Here's how the part is built. I have some questions about the finished solid (model axes, mm). A direction names the side the tool comes from. Round coordinates to 2 decimals unless told otherwise and drop trailing zeros. Order: outer loops, then holes, each group sorted by start corner. A loop starts at its lowest first (then second) coordinate and runs counter-clockwise, first axis right, second up. Notation, with made-up numbers: M 7.5,-3 L 28.5,-3 A10 ccw 28.5,11 Z; hole C -29,54.25 d1. An arc over 180 degrees is marked long. Write each question's results on one line, items separated by ' | '. Start each with the question number.
```python
from build123d import *

# Parameters (mm, degrees)
SKETCH1_R                 = 24
BOSS_EXTRUDE1_DEPTH       = 3.8
SKETCH2_R                 = 18.7
BOSS_EXTRUDE2_DEPTH       = 4.5
SKETCH3_R                 = 1
CUT_EXTRUDE1_DEPTH        = 4.5
SKETCH4_R                 = 13.6
CUT_EXTRUDE2_DEPTH        = 35.941236383
SKETCH5_R                 = 40
BOSS_EXTRUDE3_DEPTH       = 17.4
SKETCH6_R                 = 32.9
CUT_EXTRUDE6_DEPTH        = 12.4
CUT_EXTRUDE7_START        = -12.4
SKETCH7_R                 = 13.6
CUT_EXTRUDE7_DEPTH        = 12.4
M2X0_4_TAPPED_HOLE1_D     = 1.6
M2X0_4_TAPPED_HOLE1_DEPTH = 5
M2X0_4_TAPPED_HOLE1_TIP   = 0.480688495


with BuildPart() as part:
    # Sketch1 → Boss-Extrude1 (new body)
    with BuildSketch(Plane.XY):
        with Locations(Location((0, 0, 0), (0, 0, 180))):
            Circle(SKETCH1_R)
    extrude(amount=BOSS_EXTRUDE1_DEPTH)

    # Sketch2 → Boss-Extrude2 (add)
    with BuildSketch(Plane.XY.offset(3.8)):
        Circle(SKETCH2_R)
    extrude(amount=BOSS_EXTRUDE2_DEPTH)

    # Sketch3 → Cut-Extrude1 (cut)
    with BuildSketch(Plane.XY.offset(3.8)):
        with Locations((0, 22.2)):
            Circle(SKETCH3_R)
    extrude(amount=-CUT_EXTRUDE1_DEPTH, mode=Mode.SUBTRACT)

    # Sketch4 → Cut-Extrude2 (cut, through all)
    with BuildSketch(Plane.XY.offset(8.3)):
        Circle(SKETCH4_R)
    extrude(amount=-CUT_EXTRUDE2_DEPTH, mode=Mode.SUBTRACT)

    # Sketch5 → Boss-Extrude3 (add)
    with BuildSketch(Plane.XY.offset(8.3)):
        Circle(SKETCH5_R)
    extrude(amount=BOSS_EXTRUDE3_DEPTH)

    # Sketch6 → Cut-Extrude6 (cut)
    with BuildSketch(Plane.XY.offset(25.7)):
        Circle(SKETCH6_R)
    extrude(amount=-CUT_EXTRUDE6_DEPTH, mode=Mode.SUBTRACT)

    # Sketch7 → Cut-Extrude7 (cut)
    with BuildSketch(Plane(origin=(0, 0, 8.3), x_dir=(-1, 0, 0), z_dir=(0, 0, -1)).offset(CUT_EXTRUDE7_START)):
        with Locations(Location((0, 0, 0), (0, 0, 180))):
            Circle(SKETCH7_R)
    extrude(amount=CUT_EXTRUDE7_DEPTH, mode=Mode.SUBTRACT)

    # M2x0.4 Tapped Hole1
    with Locations(Plane(origin=(0, 36.45, 25.7), x_dir=(1, 0, 0), z_dir=(0, 0, 1))):
        with Locations((0, 0), (-31.566625968, -54.6), (31.501674063, -54.6375)):
            Hole(M2X0_4_TAPPED_HOLE1_D / 2, depth=M2X0_4_TAPPED_HOLE1_DEPTH)
            with Locations((0, 0, -(M2X0_4_TAPPED_HOLE1_DEPTH + M2X0_4_TAPPED_HOLE1_TIP / 2))):  # 118° drill point
                Cone(0, M2X0_4_TAPPED_HOLE1_D / 2, M2X0_4_TAPPED_HOLE1_TIP, mode=Mode.SUBTRACT)


solid = part.part
```
(1) If we mould it in two halves opening along Z, with no side actions, what happens to faces 1 (the cylindrical face through (-4.054, -18.255, 6.018)), 2 (the cylindrical face through (-7.13, -32.12, 19.59)), 3 (the flat face through (-3, 33, 25.7))? For each: pulls with the +Z half, pulls with the -Z half, needs draft (parallel to the pull), parting line crosses it, or undercut.
(2) I want a section at D-D on z = 12. Write out the boundary of the cut face in (x, y), and give its area (3 significant figures).
(3) Please list where these lines run through material, in increasing order: line 1 (Y direction, x = 0, z = 2.25); line 2 (Y direction, x = 0, z = 23.1); line 3 (Z direction, x = -5, y = 22).
(4) I'm going to push flat-ended pins straight in: pin 1 Ø12 at (x, y) = (-16, -4.5) entering from +Z; pin 2 Ø8 at (y, z) = (-23.5, 11) entering from -X; pin 3 Ø1 at (x, z) = (-6.5, 8) entering from -Y; pin 4 Ø24.5 at (x, y) = (0, 0) entering from +Z. Where does each tip first touch, or does it pass through?
(5) I want a section at C-C on y = 22.2. Write out the boundary of the cut face in (x, z).
(6) I want a section at A-A on y = 0. Write out the boundary of the cut face in (x, z).
(7) On a 3-axis mill with a long thin cutter (end or side, diameter ignored), from which of +Z, -Z, +X, -X, +Y, -Y can I reach the whole of each face in a straight line? I mean faces 4 (the flat face through (-10, 10, 0)), 5 (the flat face through (14, 0, 13.3)), 6 (the flat face through (8.3, -17.2, 8.3)), 7 (the cylindrical face through (0.46, 21.31, 1.93)), 8 (the cylindrical face through (-8.67, -39.05, 16.88)). Say none if no direction works.
(8) I want a section at B-B on x = -20.5. Write out the boundary of the cut face in (y, z).
Solutions:
1) face 1: undercut | face 2: needs draft | face 3: pulls with the +Z half
2) outline: C 0,0 d80; hole C 0,0 d27.2 | area: 4,450 mm^2
3) line 1: -24 to -13.6, 13.6 to 21.2, 23.2 to 24 | line 2: -40 to -32.9, 32.9 to 35.65, 37.25 to 40 | line 3: 0 to 3.8, 8.3 to 13.3
4) pin 1: z = 13.3 | pin 2: x = -34.92 | pin 3: y = -39.53 | pin 4: through
5) outline: M -33.27,8.3 L 33.27,8.3 L 33.27,25.7 L 24.28,25.7 L 24.28,13.3 L -24.28,13.3 L -24.28,25.7 L -33.27,25.7 Z; M -9.12,0 L -1,0 L -1,3.8 L -9.12,3.8 Z; M 1,0 L 9.12,0 L 9.12,3.8 L 1,3.8 Z
6) outline: M -40,8.3 L -18.7,8.3 L -18.7,3.8 L -24,3.8 L -24,0 L -13.6,0 L -13.6,13.3 L -32.9,13.3 L -32.9,25.7 L -40,25.7 Z; M 13.6,0 L 24,0 L 24,3.8 L 18.7,3.8 L 18.7,8.3 L 40,8.3 L 40,25.7 L 32.9,25.7 L 32.9,13.3 L 13.6,13.3 Z
7) face 4: -Z, +X, -X, +Y, -Y | face 5: +Z | face 6: none | face 7: -Z | face 8: +Z, -Z
8) outline: M -34.35,8.3 L 34.35,8.3 L 34.35,25.7 L 25.73,25.7 L 25.73,13.3 L -25.73,13.3 L -25.73,25.7 L -34.35,25.7 Z; M -12.48,0 L 12.48,0 L 12.48,3.8 L -12.48,3.8 Z
